Build history of the part. All positions in model axes, mm. Face numbers are marked on the shaded views. A direction names the side the tool comes from. Round coordinates to 2 decimals unless told otherwise and drop trailing zeros. Write each loop counter-clockwise with the first axis right and the second up, starting at its lowest first coordinate (ties: lowest second). Pieces come first, ordered by that corner, then holes. Notation, with made-up numbers: (4.5, -37) - (18.5, -37) arc R36 ccw to (18.5, -2) - close; hole circle Ø8 at (45.5, 38.5). An arc over 180 degrees is marked (long way). Write each question's results on one line, items separated by ' | '.
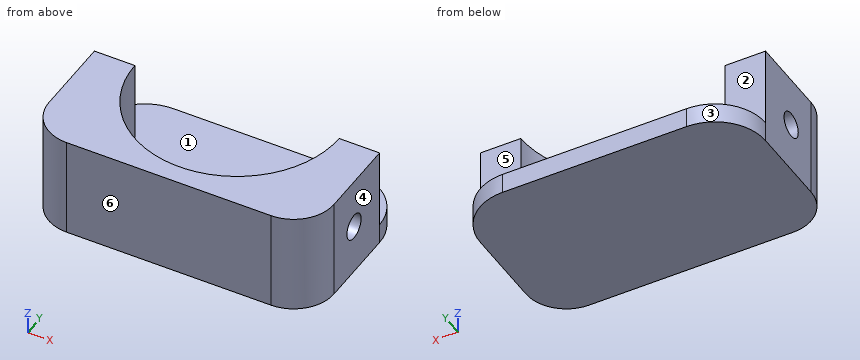
from build123d import *

# Parameters (mm, degrees)
EXTRUDE_1_DEPTH     = 8
EXTRUDE_2_DEPTH     = 2
SKETCH_3_R          = 1.25
CUT_EXTRUDE_1_DEPTH = 32.673964071
FILLET_1_R          = 5
FILLET_2_R          = 4


with BuildPart() as part:
    # 草图1 → 凸台-拉伸1 (new body)
    with BuildSketch(Plane.XY):
        with BuildLine():
            Line((-10.1, 0), (-14.1, 0))
            Line((-14.1, 0), (-14.1, -12))
            Line((-14.1, -12), (14.1, -12))
            Line((14.1, -12), (14.1, 0))
            Line((14.1, 0), (10.1, 0))
            ThreePointArc((10.1, 0), (0, -10.1), (-10.1, 0))
        make_face()
    extrude(amount=EXTRUDE_1_DEPTH)

    # 草图2 → 凸台-拉伸2 (add)
    with BuildSketch(Plane(origin=(0, 0, 0), x_dir=(-1, 0, 0), z_dir=(0, 0, -1))):
        with BuildLine():
            Line((-14.1, -12), (-14.1, 0))
            ThreePointArc((-14.1, 0), (-13.869033835, 2.541633427), (-13.18370206, 5))
            Line((-13.18370206, 5), (13.18370206, 5))
            ThreePointArc((13.18370206, 5), (13.869033835, 2.541633427), (14.1, 0))
            Line((14.1, 0), (14.1, -12))
            Line((14.1, -12), (-14.1, -12))
        make_face()
    extrude(amount=EXTRUDE_2_DEPTH)

    # 草图3 → 切除-拉伸1 (cut, through all)
    with BuildSketch(Plane.ZY.offset(14.1)):
        with Locations(Location((3, -4.5, 0), (0, 0, 270))):
            Circle(SKETCH_3_R)
    extrude(amount=-CUT_EXTRUDE_1_DEPTH, mode=Mode.SUBTRACT)

    # 圆角1
    fillet_1_edges = [part.edges().sort_by_distance(p)[0] for p in [
        (-13.18370206, 5, -1),
        (13.18370206, 5, -1),
    ]]
    fillet(fillet_1_edges, radius=FILLET_1_R - 0.0001)  # a hair under: the kernel refuses the full size

    # 圆角2
    fillet_2_edges = [part.edges().sort_by_distance(p)[0] for p in [
        (14.1, -12, 3),
        (-14.1, -12, 3),
    ]]
    fillet(fillet_2_edges, radius=FILLET_2_R)


solid = part.part
(1) Tool access for the marked faces 5 and 6: list every direction of +Z, -Z, +X, -X, +Y, -Y with a clear straight run to the whole face (end or side of a thin tool).
Worked answers:
face 5: +Z, +X, -X, +Y | face 6: +Z, -Z, +X, -X, -Y
(2) Slice it at C-C, the plane z = 3. Write the cut outline in (x, y).
Worked answers:
outline: (-14.1, -8) arc R4 ccw to (-10.1, -12) - (10.1, -12) arc R4 ccw to (14.1, -8) - (14.1, -5.75) - (8.3, -5.75) arc R10.1 cw to (-8.3, -5.75) - (-14.1, -5.75) - close; (-14.1, -3.25) - (-9.56, -3.25) arc R10.1 cw to (-10.1, 0) - (-14.1, 0) - close; (9.56, -3.25) - (14.1, -3.25) - (14.1, 0) - (10.1, 0) arc R10.1 cw to start
(3) Two-plate mould, pull along X, no slides. Class the marked faces 1, 2, 3 and 4: released by +X, released by -X, zero draft, split by the parting line, or undercut.
Worked answers:
face 1: undercut | face 2: zero draft | face 3: released by -X | face 4: released by +X
(4) Slice it at B-B, the plane x = -5.75. Write the cut outline in (y, z).
Worked answers:
outline: (-12, -2) - (5, -2) - (5, 0) - (-8.3, 0) - (-8.3, 8) - (-12, 8) - close
(5) Slice it at A-A, the plane z = 0.5. Write the cut outline in (x, y), and give its area (3 significant figures).
Worked answers:
outline: (-14.1, -8) arc R4 ccw to (-10.1, -12) - (10.1, -12) arc R4 ccw to (14.1, -8) - (14.1, 0) - (10.1, 0) arc R10.1 cw to (-10.1, 0) - (-14.1, 0) - close | area: 171 mm2
(6) Flat gauge pins, fed straight in: pin 1 Ø3 at (x, z) = (12, 2.5) entering from +Y; pin 2 Ø1 at (x, y) = (3, 3.5) entering from +Z. Where does each tip first touch, or does it go through?
Worked answers:
pin 1: stops at y = 0 | pin 2: stops at z = 0
(7) Slice it at D-D, the plane y = -6.25. Write the cut outline in (x, z), and give its area (3 significant figures).
Worked answers:
outline: (-14.1, -2) - (14.1, -2) - (14.1, 8) - (7.93, 8) - (7.93, 0) - (-7.93, 0) - (-7.93, 8) - (-14.1, 8) - close | area: 155 mm2
(8) Drill centre lines: probe 1 along Z at (x, y) = (-10.2, -4.5); probe 2 along Y at (x, z) = (11.4, 3); probe 3 along X at (y, z) = (-6.25, 1.5). Where is each one in solid material? Low to high. Write a range as [from, to].
Worked answers:
probe 1: z = [-2, 1.75], [4.25, 8] | probe 2: y = [-11.78, -5.75], [-3.25, 0] | probe 3: x = [-14.1, -7.93], [7.93, 14.1]
